Work out the finished part from the listing and answer in its coordinate system (mm). A direction names the side the tool comes from. Give positions to 0.01 mm unless a question says otherwise; leave off trailing zeros. Order: outer loops, then holes, each group sorted by start corner. A loop starts at its lowest first (then second) coordinate and runs counter-clockwise, first axis right, second up.
```python
from build123d import *

# Parameters (mm, degrees)
F0_W     = 145
F0_H     = 10.5
F1_DEPTH = 36
F2_R     = 5
F3_T     = 5
F4_R     = 5


# Not quite as in the source:
# - a shell that OpenCascade refuses in one call is made with other operations: the cavity is built on its own and cut out


with BuildPart() as f1:
    # F0 (on Right) → F1 (new body, symmetric)
    with BuildSketch(Plane.YZ):
        Rectangle(F0_W, F0_H)
    extrude(amount=F1_DEPTH, both=True)

    # F2
    f2_edges = [f1.edges().sort_by_distance(p)[0] for p in [
        (36, -72.5, 0),
        (36, 72.5, 0),
        (-36, -72.5, 0),
        (-36, 72.5, 0),
    ]]
    fillet(f2_edges, radius=F2_R)

    # F3: shell of thickness 5, made by hand


with BuildPart() as f3_core1:
    # F3_t2: copy of F1
    add(f1.part)

    # the walls: a layer under each face that stays
    f3_faces = [f3_core1.faces().sort_by_distance(p)[0] for p in [
        (-36, 0, 0),
        (0, -72.5, 0),
        (0, 72.5, 0),
        (36, 0, 0),
        (0, 0, 5.25),
    ]]
    thicken(f3_faces, amount=-F3_T, mode=Mode.SUBTRACT)


with BuildPart() as f1_1:
    add(f1.part)

    # what is left inside the walls is the cavity
    f3_cavity = [f3_core1.part.solids().sort_by_distance(p)[0] for p in [
        (-10.333333, 0, -5.2),
    ]]
    add(f3_cavity, mode=Mode.SUBTRACT)

    # F4
    f4_edges = [f1_1.edges().sort_by_distance(p)[0] for p in [
        (-31, -67.5, -2.5),
        (31, -67.5, -2.5),
        (-31, 67.5, -2.5),
        (31, 67.5, -2.5),
    ]]
    fillet(f4_edges, radius=F4_R)


solid = f1_1.part
```
1. The part is cut by section C-C (x = 16). Write down the section's boundary in (y, z).
Findings below:
outline: (-72.5, -5.25) - (-67.5, -5.25) - (-67.5, 0.25) - (67.5, 0.25) - (67.5, -5.25) - (72.5, -5.25) - (72.5, 5.25) - (-72.5, 5.25) - close
2. The part is cut by section A-A (z = -3.5). Write down the section's boundary in (x, y), then the cut area to 3 significant figures.
Findings below:
outline: (-36, -67.5) arc R5 ccw to (-31, -72.5) - (31, -72.5) arc R5 ccw to (36, -67.5) - (36, 67.5) arc R5 ccw to (31, 72.5) - (-31, 72.5) arc R5 ccw to (-36, 67.5) - close; hole (-31, -62.5) arc R5 ccw to (-26, -67.5) - (26, -67.5) arc R5 ccw to (31, -62.5) - (31, 62.5) arc R5 ccw to (26, 67.5) - (-26, 67.5) arc R5 ccw to (-31, 62.5) - close
area: 2,070 mm2
3. The mould has two halves that part along X. Classify faces 3 (the face through (-31, -1, -2)), 4 (the face through (1, -1, 5.25)), 5 (the face through (34.5, -71.07, 0.07)), 6 (the face through (31, -1, -2)): pulls with the +X half, pulls with the -X half, needs draft (parallel to the pull), parting line crosses it, or undercut.
Findings below:
face 3: undercut
face 4: needs draft
face 5: pulls with the +X half
face 6: undercut
4. Straight lines are drawn through the part: probe 1 along Y at (x, z) = (-20.5, -3); probe 2 along X at (y, z) = (40.5, -3.5); probe 3 along Z at (x, y) = (-11, 26). For each, find the intervals that lie inside material, in ascending order.
Findings below:
probe 1: y = -72.5 to -67.5, 67.5 to 72.5
probe 2: x = -36 to -31, 31 to 36
probe 3: z = 0.25 to 5.25
5. Given P1, Ø8, axis at x = 18.5, y = 4.5, coming from the -Z side, flat-ended and moving along its own axis, determine where the tip first touches the part or whether it passes through.
Findings below:
P1: stops at z = 0.25
6. Which of the six approach directions +Z, -Z, +X, -X, +Y, -Y give full straight-line access (tool end or side, diameter ignored) to faces 1 (the face through (0, -72.5, 0)), 2 (the face through (-29.57, -66, -2.46))?
Findings below:
face 1: +Z, -Z, +X, -X, -Y
face 2: -Z
7. The part is cut by section B-B (y = -24). Write down the section's boundary in (x, z).
Findings below:
outline: (-36, -5.25) - (-31, -5.25) - (-31, 0.25) - (31, 0.25) - (31, -5.25) - (36, -5.25) - (36, 5.25) - (-36, 5.25) - close
